Can you work these out from the drawing? Everything is in mm from the part's minimum corner. Round coordinates to 2 decimals unless told otherwise and drop trailing zeros. Loops run counter-clockwise (first coordinate to the right, second up) from the corner with the lowest first, then second, coordinate; pieces in that order, holes last. Notation, with made-up numbers: (6, -3.5) -> (30, -3.5) arc R35 cw to (30, 32.5) -> close; hole circle Ø9 at (49.25, 67). An arc over 180 degrees is marked (long way). One line per item, written item: value.
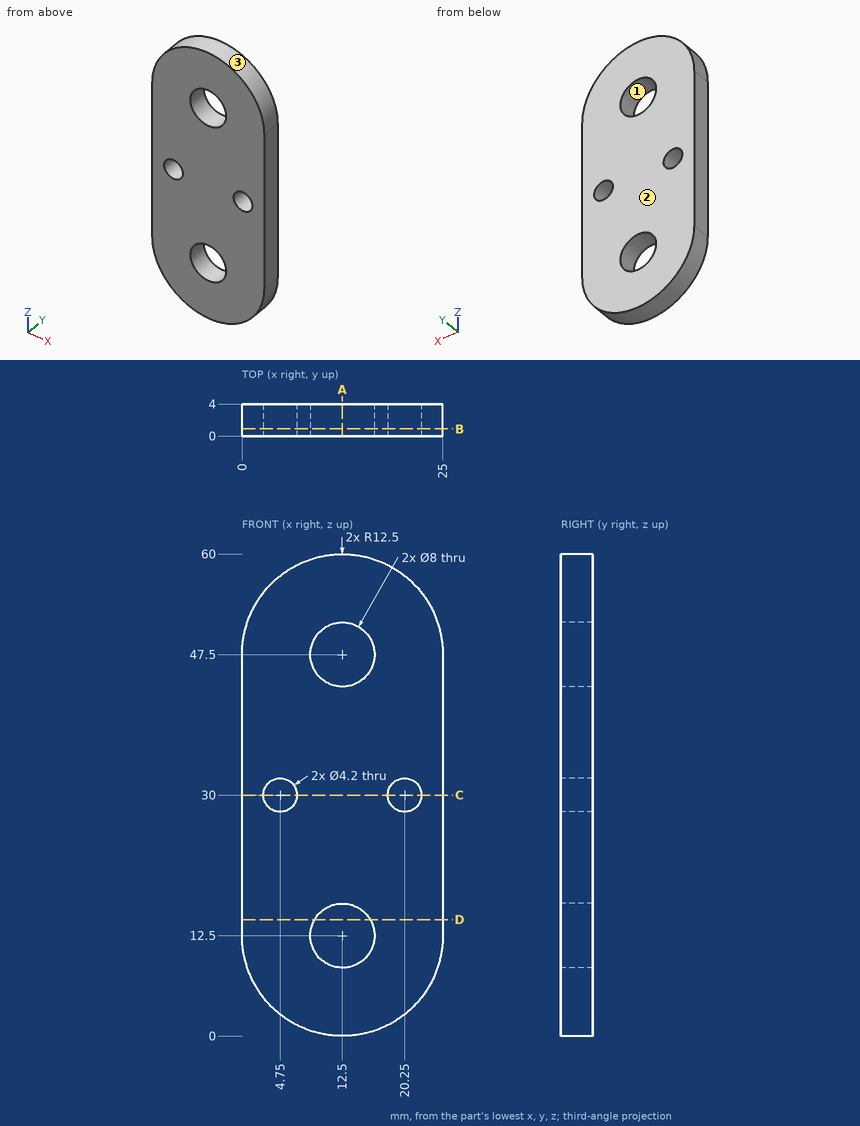
Item 1: I need wall thicknesses on line 1 (X direction, y = 1.7, z = 30); line 2 (Z direction, x = 12.5, y = 1.45); line 3 (X direction, y = 1.15, z = 47.5). Which ranges of each line are inside material? Lowest first, please. Write a range as from..to.
Output:
line 1: x = 0..2.65, 6.85..18.15, 22.35..25
line 2: z = 0..8.5, 16.5..43.5, 51.5..60
line 3: x = 0..8.5, 16.5..25
Item 2: If we section it at C-C on z = 30: List the corners of the cut face in (x, y) for me.
Output:
outline: (0, 0) -> (2.65, 0) -> (2.65, 4) -> (0, 4) -> close; (6.85, 0) -> (18.15, 0) -> (18.15, 4) -> (6.85, 4) -> close; (22.35, 0) -> (25, 0) -> (25, 4) -> (22.35, 4) -> close
Item 3: Will these pins go through, and if not, where does the flat tip stop? pin 1 Ø2 at (y, z) = (0.5, 51) entering from -X; pin 2 Ø2 at (x, y) = (7.5, 2) entering from +Z; pin 3 Ø1 at (x, y) = (9.5, 3) entering from +Z.
Output:
pin 1: stops at x = 0.25
pin 2: stops at z = 59.34
pin 3: stops at z = 59.75
Item 4: If we section it at D-D on z = 14.5: List the corners of the cut face in (x, y) for me, plus the area to 3 significant figures.
Output:
outline: (0, 0) -> (9.04, 0) -> (9.04, 4) -> (0, 4) -> close; (15.96, 0) -> (25, 0) -> (25, 4) -> (15.96, 4) -> close
area: 72.3 mm²
Item 5: If we section it at B-B on y = 0.9: List the corners of the cut face in (x, z) for me, plus the area to 3 significant figures.
Output:
outline: (0, 12.5) arc R12.5 ccw to (25, 12.5) -> (25, 47.5) arc R12.5 ccw to (0, 47.5) -> close; hole circle Ø4.2 at (4.75, 30); hole circle Ø8 at (12.5, 12.5); hole circle Ø8 at (12.5, 47.5); hole circle Ø4.2 at (20.25, 30)
area: 1,240 mm²
Item 6: If we section it at A-A on x = 12.5: List the corners of the cut face in (y, z) for me, plus the area to 3 significant figures.
Output:
outline: (0, 0) -> (4, 0) -> (4, 8.5) -> (0, 8.5) -> close; (0, 16.5) -> (4, 16.5) -> (4, 43.5) -> (0, 43.5) -> close; (0, 51.5) -> (4, 51.5) -> (4, 60) -> (0, 60) -> close
area: 176 mm²
Item 7: If we mould it in two halves opening along Z, with no side actions, what happens to the marked faces 1, 2 and 3? For each: released by +Z, released by -Z, zero draft, split by the parting line, or undercut.
Output:
face 1: undercut
face 2: zero draft
face 3: released by +Z
